from build123d import *

# Parameters (mm, degrees)
F1_DEPTH = 2
F0_W     = 142
F0_H     = 143
F2_DEPTH = 38
F0_W_2   = 154
F0_H_2   = 27
F3_DEPTH = 35


with BuildPart() as f1:
    # F0 (on Top) → F1 (new body)
    with BuildSketch(Plane.XY):
        Polygon((152.5, 122.5), (-152.5, 122.5), (-152.5, 79.5), (-10.5, 79.5), (-10.5, -63.5), (-152.5, -63.5), (-152.5, -95.5), (1.5, -95.5), (1.5, -122.5), (152.5, -122.5), align=None)
    extrude(amount=F1_DEPTH)

    # F0 (on Top) → F2 (join)
    with BuildSketch(Plane.XY):
        with Locations((-81.5, 8)):
            Rectangle(F0_W, F0_H)
    extrude(amount=F2_DEPTH)

    # F0 (on Top) → F3 (join)
    with BuildSketch(Plane.XY):
        with Locations((-75.5, -109)):
            Rectangle(F0_W_2, F0_H_2)
    extrude(amount=F3_DEPTH)


solid = f1.part
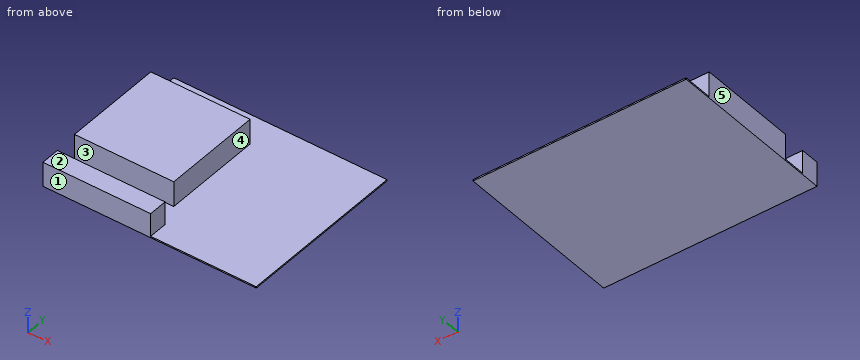
Source: CAD feature listing. Evaluate the final solid. Frame: model axes, mm. Face numbers are marked on the shaded views. A direction names the side the tool comes from. Round coordinates to 2 decimals unless told otherwise and drop trailing zeros. Loops run counter-clockwise (first coordinate to the right, second up) from the corner with the lowest first, then second, coordinate; pieces in that order, holes last. Notation, with made-up numbers: M 11.25,4 L 30.25,4 A15 ccw 30.25,33 Z; hole C 52.5,17 d1. An arc over 180 degrees is marked long. Return JSON: item names as keys, results as strings. Group by question number.
1. Section query C-C on x = -126.5. Output: boundary loops of the cut face in (y, z).
2. Pin query (flat end, axial travel): pin 1 (4 mm diameter, centred on y = 29, z = 30, fed in from +X); pin 2 (8 mm diameter, centred on x = -63.5, z = 24, fed in from +Y); pin 3 (13.5 mm diameter, centred on y = -105.5, z = 19.5, fed in from +X). Return the tip coordinate at first contact, or that it passes through.
3. Section query B-B on y = 22. Output: boundary loops of the cut face in (x, z), and give its area (3 significant figures).
4. Reachability of the marked faces 4 and 5 from +Z, -Z, +X, -X, +Y, -Y: full face, straight path, thin tool, end or side. Return the list, or none.
5. Mould query, pull axis Y, two halves, no side actions, for the marked faces 1, 2 and 3. Classes: released by +Y, released by -Y, zero draft, split by the parting line, or undercut.
6. Section query A-A on z = 23.5. Output: boundary loops of the cut face in (x, y).
7. Section query D-D on y = -104.5. Output: boundary loops of the cut face in (x, z).
8. Material intervals for line 1 along Y through (x, z) = (-108, 2.5); line 2 along X through (y, z) = (-110, 6.5); line 3 along Y through (x, z) = (-1, 17), sorted ascending. Write a range as from..to.
Checks:
{
 "1": {"outline": "M -122.5,0 L 122.5,0 L 122.5,2 L 79.5,2 L 79.5,38 L -63.5,38 L -63.5,2 L -95.5,2 L -95.5,35 L -122.5,35 Z"},
 "2": {"pin 1": "stops at x = -10.5", "pin 2": "stops at y = 79.5", "pin 3": "stops at x = 1.5"},
 "3": {"outline": "M -152.5,0 L 152.5,0 L 152.5,2 L -10.5,2 L -10.5,38 L -152.5,38 Z", "area": "5,720 mm²"},
 "4": {"face 4": "+Z, +X, +Y", "face 5": "+Z, -Z, -X, +Y, -Y"},
 "5": {"face 1": "released by -Y", "face 2": "zero draft", "face 3": "undercut"},
 "6": {"outline": "M -152.5,-122.5 L 1.5,-122.5 L 1.5,-95.5 L -152.5,-95.5 Z; M -152.5,-63.5 L -10.5,-63.5 L -10.5,79.5 L -152.5,79.5 Z"},
 "7": {"outline": "M -152.5,0 L 152.5,0 L 152.5,2 L 1.5,2 L 1.5,35 L -152.5,35 Z"},
 "8": {"line 1": "y = -122.5..-95.5, -63.5..79.5", "line 2": "x = -152.5..1.5", "line 3": "y = -122.5..-95.5"}
}
